```python
from build123d import *

# Parameters (mm, degrees)
BOSS_EXTRUDE1_DEPTH = 4


with BuildPart() as part:
    # Sketch1 → Boss-Extrude1 (new body)
    with BuildSketch(Plane.XY):
        with BuildLine():
            ThreePointArc((0, 4.7), (3.323401872, 3.323401872), (4.7, 0))
            ThreePointArc((4.7, 0), (3.323401872, -3.323401872), (0, -4.7))
            Line((0, -4.7), (0, -14.1))
            ThreePointArc((0, -14.1), (9.970205615, -9.970205615), (14.1, 0))
            ThreePointArc((14.1, 0), (11.512601791, 8.140638796), (4.7, 13.293607486))
            ThreePointArc((4.7, 13.293607486), (3.538135112, 13.648868082), (2.35, 13.90278749))
            ThreePointArc((2.35, 13.90278749), (1.17913027, 14.050610371), (0, 14.1))
            Line((0, 14.1), (0, 4.7))
        make_face()
        with BuildLine():
            Line((0, -14.1), (0, -4.7))
            ThreePointArc((0, -4.7), (-4.7, 0), (0, 4.7))
            Line((0, 4.7), (0, 14.1))
            ThreePointArc((0, 14.1), (-1.17913027, 14.050610371), (-2.35, 13.90278749))
            ThreePointArc((-2.35, 13.90278749), (-3.538135112, 13.648868082), (-4.7, 13.293607486))
            ThreePointArc((-4.7, 13.293607486), (-13.896939691, -2.3843379), (0, -14.1))
        make_face()
        with BuildLine():
            ThreePointArc((-2.35, 13.90278749), (-1.17913027, 14.050610371), (0, 14.1))
            Line((0, 14.1), (0, 65.9))
            Line((0, 65.9), (-2.35, 65.9))
            Line((-2.35, 65.9), (-2.35, 55.625335767))
            ThreePointArc((-2.35, 55.625335767), (-2.402477907, 54.602201264), (-2.559360842, 53.589805153))
            Line((-2.559360842, 53.589805153), (-4.408193437, 44.697159337))
            ThreePointArc((-4.408193437, 44.697159337), (-4.597967377, 43.28721197), (-4.585741176, 41.864603012))
            Line((-4.585741176, 41.864603012), (-2.35, 13.90278749))
        make_face()
        with BuildLine():
            Line((0, 65.9), (0, 14.1))
            ThreePointArc((0, 14.1), (1.17913027, 14.050610371), (2.35, 13.90278749))
            Line((2.35, 13.90278749), (4.585741176, 41.864603012))
            ThreePointArc((4.585741176, 41.864603012), (4.597967377, 43.28721197), (4.408193437, 44.697159337))
            Line((4.408193437, 44.697159337), (2.559360842, 53.589805153))
            ThreePointArc((2.559360842, 53.589805153), (2.402477907, 54.602201264), (2.35, 55.625335767))
            Line((2.35, 55.625335767), (2.35, 65.9))
            Line((2.35, 65.9), (0, 65.9))
        make_face()
    extrude(amount=BOSS_EXTRUDE1_DEPTH)


solid = part.part
```
Check sheet for the modelled part. Datum: model origin and axes. Units: mm. A direction names the side the tool comes from. Coordinates: 2 decimals unless noted, no trailing zeros. Write each loop counter-clockwise with the first axis right and the second up, starting at its lowest first coordinate (ties: lowest second). Pieces come first, ordered by that corner, then holes. Notation, with made-up numbers: M 75.5,46.25 L 116.5,46.25 A19 cw 116.5,62.25 Z; hole C -10.5,48 d11. An arc over 180 degrees is marked long. Write item = value, one per line. Start each with the question number.
1. Tool access check on faces 1 (the flat face through (2.35, 61, 2)), 2 (the flat face through (-2.35, 61, 2)), 3 (the flat face through (-3.484, 28.079, 1.972)), 4 (the flat face through (3.452, 27.688, 1.972)), 5 (the flat face through (0, 65.9, 2)). Record the directions out of +Z, -Z, +X, -X, +Y, -Y that give a thin tool (end or side, any length) a straight path to the whole face; none if there is none.
2. Sectioned sample at B-B (y = 26.5). Record the cut outline in (x, z).
3. Sectioned sample at A-A (z = 2.05). Record the cut outline in (x, y).
4. Sectioned sample at C-C (x = -8.75). Record the cut outline in (y, z), then the cut area to 3 significant figures.
5. Go/stop test with flat-tipped pins: pin 1 (2 mm diameter, centred on y = 7, z = 0.5, fed in from +X); pin 2 (8 mm diameter, centred on x = 8.5, y = 36.5, fed in from -Z); pin 3 (2 mm diameter, centred on y = 53, z = 2.5, fed in from +X). Record where each tip stops, or that it passes through.
6. Thickness scan on probe 1 along X at (y, z) = (1.5, 3.45); probe 2 along X at (y, z) = (2.5, 2.85); probe 3 along Y at (x, z) = (-10.25, 3.6). Record the ranges inside material, lowest first.
The answers:
q1.face_1 = +Z, -Z, +X, +Y
q1.face_2 = +Z, -Z, -X, +Y
q1.face_3 = +Z, -Z, -X
q1.face_4 = +Z, -Z, +X
q1.face_5 = +Z, -Z, +X, -X, +Y
q2.outline = M -3.36,0 L 3.36,0 L 3.36,4 L -3.36,4 Z
q3.outline = M -4.59,41.86 L -2.35,13.9 A14.1 ccw long 2.35,13.9 L 4.59,41.86 A10 ccw 4.41,44.7 L 2.56,53.59 A10 cw 2.35,55.63 L 2.35,65.9 L -2.35,65.9 L -2.35,55.63 A10 cw -2.56,53.59 L -4.41,44.7 A10 ccw Z; hole C 0,0 d9.4
q4.outline = M -11.06,0 L 11.06,0 L 11.06,4 L -11.06,4 Z
q4.area = 88.5 mm²
q5.pin_1 = 12.76
q5.pin_2 = through
q5.pin_3 = 2.89
q6.probe_1 = -14.02 to -4.45, 4.45 to 14.02
q6.probe_2 = -13.88 to -3.98, 3.98 to 13.88
q6.probe_3 = -9.68 to 9.68
